Autodesk Inventor part; units mm, degrees
ref_plane "YZ Plane" through (0, 0, 0) normal (1, 0, 0) x (0, 1, 0)
ref_plane "XZ Plane" through (0, 0, 0) normal (0, 1, 0) x (-1, 0, 0)
ref_plane "XY Plane" through (0, 0, 0) normal (0, 0, 1) x (1, 0, 0)
sketch "スケッチ1" plane through (0, 0, 0) normal (0, 0, 1) x (1, 0, 0)
  circle A0 centre (0, 0) radius 5
  dimension "d0" = 10
extrude "押し出し1" add sketch "スケッチ1" along normal blind 65
sketch "スケッチ2" plane through (0, 0, 65) normal (0, 0, 1) x (1, 0, 0)
  point P0 (0, 0)
  point P1 (0, 0)
hole "穴1" at (0, 0, 65) direction (0, 0, -1) diameter 3.242 depth 15 tip angle 118
sketch "スケッチ3" plane through (0, 0, 0) normal (0, 0, -1) x (-1, 0, 0)
  circle A0 centre (0, 0) radius 1.621
hole "穴2" at (0, 0, 0) direction (0, 0, 1) diameter 3.242 depth 15 tip angle 118
properties part number "link1part3" material "アルミニウム 6061"
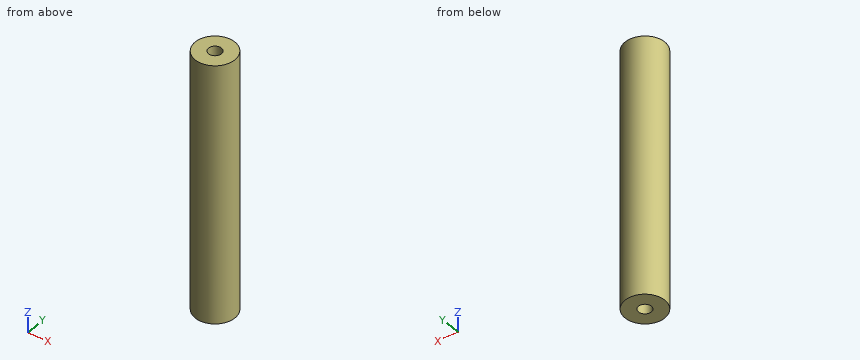
Source: CAD feature listing. Evaluate the final solid. Frame: model axes, mm. Coordinates: 2 decimals unless noted, no trailing zeros. Loops run counter-clockwise (first coordinate to the right, second up) from the corner with the lowest first, then second, coordinate; pieces in that order, holes last. Notation, with made-up numbers: M 61,-22.5 L 101,-22.5 A15 cw 101,-17.5 Z; hole C 63.5,-33.5 d7. An arc over 180 degrees is marked long. Use a Markdown table: item, result. Add a question column.
Q1. First-contact query: pin 1 (1.9 mm diameter, centred on x = 0, y = 0, fed in from -Z); pin 2 (1 mm diameter, centred on y = -3.5, z = 39, fed in from -X). Flat tips, straight axial feed; report the tip coordinate or a pass-through.
Q2. Section query B-B, the plane z = 41. Return loops of the section in (x, y).
Q3. Section query D-D, the plane x = -2.5. Return loops of the section in (y, z), and give its area (3 significant figures).
Q4. Section query C-C, the plane y = 3.25. Return loops of the section in (x, z), and give its area (3 significant figures).
Q5. Section query A-A, the plane z = 12. Return loops of the section in (x, y).
Q6. Material intervals for L1, parallel to Y at x = 0, z = 57.25; L2, parallel to X at y = 0.75, z = 8; L3, parallel to X at y = -1.25, z = 4.5, sorted ascending.
Result:
| question | item | result |
|---|---|---|
| 1 | pin 1 | stops at z = 15.4 |
| 1 | pin 2 | stops at x = -4 |
| 2 | outline | C 0,0 d10 |
| 3 | outline | M -4.33,0 L 4.33,0 L 4.33,65 L -4.33,65 Z |
| 3 | area | 563 mm2 |
| 4 | outline | M -3.8,0 L 3.8,0 L 3.8,65 L -3.8,65 Z |
| 4 | area | 494 mm2 |
| 5 | outline | C 0,0 d10; hole C 0,0 d3.24 |
| 6 | L1 | y = -5 to -1.62, 1.62 to 5 |
| 6 | L2 | x = -4.94 to -1.44, 1.44 to 4.94 |
| 6 | L3 | x = -4.84 to -1.03, 1.03 to 4.84 |
